```python
from build123d import *

# Parameters (mm, degrees)
SKETCH1_R             = 2
BOSS_EXTRUDE1_DEPTH   = 8
BOSS_EXTRUDE1_2_DEPTH = 8
BOSS_EXTRUDE2_DEPTH   = 20
BOSS_EXTRUDE3_DEPTH   = 20
BOSS_EXTRUDE4_START   = -8
SKETCH4_R             = 2
BOSS_EXTRUDE4_DEPTH   = 8
CUT_EXTRUDE1_DEPTH    = 133.91350571
SKETCH7_W             = 3
SKETCH7_H             = 9
BOSS_EXTRUDE5_DEPTH   = 20
BOSS_EXTRUDE6_DEPTH   = 3
CUT_EXTRUDE2_DEPTH    = 132.780119897
MIRROR2_COPY_1_DEPTH  = 3
MIRROR2_COPY_2_DEPTH  = 132.780119897
MIRROR3_COPY_1_DEPTH  = 3
MIRROR3_COPY_2_DEPTH  = 132.780119897
MIRROR3_COPY_3_DEPTH  = 3
MIRROR3_COPY_4_DEPTH  = 132.780119897
MIRROR3_COPY_5_DEPTH  = 3
MIRROR3_COPY_6_DEPTH  = 132.780119897


with BuildPart() as part:
    # Sketch1 → Boss-Extrude1 (new body)
    with BuildSketch(Plane.XY):
        with BuildLine():
            Line((-10, -15), (10, -15))
            ThreePointArc((10, -15), (0, -25), (-10, -15))
        make_face()
        with Locations((0, -19)):
            Circle(SKETCH1_R, mode=Mode.SUBTRACT)
    extrude(amount=-BOSS_EXTRUDE1_DEPTH)



with BuildPart() as body_2:
    # Sketch1 → Boss-Extrude1 2 (new body)
    with BuildSketch(Plane.XY):
        with BuildLine():
            Line((10, 0), (-10, 0))
            ThreePointArc((-10, 0), (0, 10), (10, 0))
        make_face()
        with Locations((0, 4)):
            Circle(SKETCH1_R, mode=Mode.SUBTRACT)
    extrude(amount=-BOSS_EXTRUDE1_2_DEPTH)


with BuildPart() as part_1:
    add(part.part)

    add(body_2.part)  # Boss-Extrude2 merges body 2
    # Sketch2 → Boss-Extrude2 (add)
    with BuildSketch(Plane.ZY.offset(10)):
        Polygon((0, -15), (67, -15), (67, -7.5), (54, -7.5), (54, 0), (0, 0), (-8, 0), (-8, -15), align=None)
    extrude(amount=-BOSS_EXTRUDE2_DEPTH)

    # Sketch3 → Boss-Extrude3 (add)
    with BuildSketch(Plane.ZY.offset(10)):
        Polygon((54, 0), (54, -7.5), (67, -7.5), (67, -15), (121, -15), (129, -15), (129, 0), (121, 0), align=None)
    extrude(amount=-BOSS_EXTRUDE3_DEPTH)

    # Sketch4 → Boss-Extrude4 (add)
    # profile 1 of 2: a face of its own
    with BuildSketch(Plane(origin=(0, 0, 121), x_dir=(-1, 0, 0), z_dir=(0, 0, -1)).offset(BOSS_EXTRUDE4_START)):
        with BuildLine():
            Line((-10, 0), (10, 0))
            ThreePointArc((10, 0), (0, 10), (-10, 0))
        make_face()
        with Locations(Location((0, 4, 0), (0, 0, 180))):
            Circle(SKETCH4_R, mode=Mode.SUBTRACT)
    # profile 2 of 2: a face of its own
    with BuildSketch(Plane(origin=(0, 0, 121), x_dir=(-1, 0, 0), z_dir=(0, 0, -1)).offset(BOSS_EXTRUDE4_START)):
        with BuildLine():
            Line((10, -15), (-10, -15))
            ThreePointArc((-10, -15), (0, -25), (10, -15))
        make_face()
        with Locations(Location((0, -19, 0), (0, 0, 180))):
            Circle(SKETCH4_R, mode=Mode.SUBTRACT)
    extrude(amount=BOSS_EXTRUDE4_DEPTH)

    # Sketch6 → Cut-Extrude1 (cut, through all)
    with BuildSketch(Plane(origin=(10, 0, 0), x_dir=(0, 0, -1), z_dir=(1, 0, 0))):
        Polygon((0, -3), (-121, -3), (-126, -3), (-126, -12), (-121, -12), (0, -12), (5, -12), (5, -3), align=None)
    extrude(amount=-CUT_EXTRUDE1_DEPTH, mode=Mode.SUBTRACT)

    # Sketch7 → Boss-Extrude5 (add)
    with BuildSketch(Plane(origin=(10, 0, 0), x_dir=(0, 0, -1), z_dir=(1, 0, 0))):
        Polygon((5, -12), (-8.403331864, -3), (-8.403331864, -4.806786238), (2.309227161, -12), align=None)
        Polygon((-5.712559024, -3), (-8.403331864, -3), (5, -12), (5, -10.193213762), align=None)
        Polygon((-11.403331864, -3), (-11.403331864, -12), (-8.403331864, -12), (-8.403331864, -4.806786238), (-8.403331864, -3), align=None)
        Polygon((-30.703894148, -3), (-37.802498898, -3), (-18.501936613, -12), (-11.403331864, -12), align=None)
        with Locations((-39.302498898, -7.5)):
            Rectangle(SKETCH7_W, SKETCH7_H)
        Polygon((-60.103061182, -3), (-67.201665932, -3), (-47.901103647, -12), (-40.802498898, -12), align=None)
        with Locations((-68.701665932, -7.5)):
            Rectangle(SKETCH7_W, SKETCH7_H)
        Polygon((-89.502228216, -3), (-96.600832966, -3), (-77.300270681, -12), (-70.201665932, -12), align=None)
        with Locations((-98.100832966, -7.5)):
            Rectangle(SKETCH7_W, SKETCH7_H)
        Polygon((-118.901395251, -3), (-126, -3), (-106.699437715, -12), (-99.600832966, -12), align=None)
    extrude(amount=-BOSS_EXTRUDE5_DEPTH)

    # Sketch9 → Boss-Extrude6 (add)
    with BuildSketch(Plane(origin=(5, 0, 0), x_dir=(0, 0, -1), z_dir=(1, 0, 0))):
        Polygon((0, -15), (0, -23.702060424), (-15, -15), align=None)
    boss_extrude6 = extrude(amount=BOSS_EXTRUDE6_DEPTH)

    # Sketch10 → Cut-Extrude2 (cut, through all)
    with BuildSketch(Plane(origin=(0, 0, 0), x_dir=(-1, 0, 0), z_dir=(0, 0, -1))):
        with BuildLine():
            Line((-8, -21), (-8, -23.702060424))
            Line((-8, -23.702060424), (-5, -23.702060424))
            Line((-5, -23.702060424), (-5, -23.660254038))
            ThreePointArc((-5, -23.660254038), (-6.634699532, -22.482029278), (-8, -21))
        make_face()
    cut_extrude2 = extrude(amount=-CUT_EXTRUDE2_DEPTH, mode=Mode.SUBTRACT)

    # Mirror1: Boss-Extrude6, Cut-Extrude2 across plane
    add(boss_extrude6.mirror(Plane(origin=(0, 0, 0), x_dir=(0, 0, 1), z_dir=(1, 0, 0))))
    add(cut_extrude2.mirror(Plane(origin=(0, 0, 0), x_dir=(0, 0, 1), z_dir=(1, 0, 0))), mode=Mode.SUBTRACT)

    # Mirror2: Boss-Extrude6, Cut-Extrude2 across plane
    add(boss_extrude6.mirror(Plane(origin=(0, 0, 60.5), x_dir=(1, 0, 0), z_dir=(0, 0, -1))))
    add(cut_extrude2.mirror(Plane(origin=(0, 0, 60.5), x_dir=(1, 0, 0), z_dir=(0, 0, -1))), mode=Mode.SUBTRACT)

    # Mirror2 copy 1 sketch → Mirror2 copy 1 (add)
    with BuildSketch(Plane(origin=(-5, 0, 121), x_dir=(0, 0, 1), z_dir=(-1, 0, 0))):
        Polygon((0, -15), (0, -23.702060424), (-15, -15), align=None)
    extrude(amount=MIRROR2_COPY_1_DEPTH)

    # Mirror2 copy 2 sketch → Mirror2 copy 2 (cut, through all)
    with BuildSketch(Plane.XY.offset(121)):
        with BuildLine():
            Line((-8, -21), (-8, -23.702060424))
            Line((-8, -23.702060424), (-5, -23.702060424))
            Line((-5, -23.702060424), (-5, -23.660254038))
            ThreePointArc((-5, -23.660254038), (-6.634699532, -22.482029278), (-8, -21))
        make_face()
    extrude(amount=-MIRROR2_COPY_2_DEPTH, mode=Mode.SUBTRACT)

    # Mirror3: Boss-Extrude6, Cut-Extrude2 across plane
    add(boss_extrude6.mirror(Plane.ZX.offset(-7.5)))
    add(cut_extrude2.mirror(Plane.ZX.offset(-7.5)), mode=Mode.SUBTRACT)

    # Mirror3 copy 1 sketch → Mirror3 copy 1 (add)
    with BuildSketch(Plane(origin=(-5, -15, 0), x_dir=(0, 0, -1), z_dir=(-1, 0, 0))):
        Polygon((0, -15), (0, -23.702060424), (-15, -15), align=None)
    extrude(amount=MIRROR3_COPY_1_DEPTH)

    # Mirror3 copy 2 sketch → Mirror3 copy 2 (cut, through all)
    with BuildSketch(Plane(origin=(0, -15, 0), x_dir=(1, 0, 0), z_dir=(0, 0, -1))):
        with BuildLine():
            Line((-8, -21), (-8, -23.702060424))
            Line((-8, -23.702060424), (-5, -23.702060424))
            Line((-5, -23.702060424), (-5, -23.660254038))
            ThreePointArc((-5, -23.660254038), (-6.634699532, -22.482029278), (-8, -21))
        make_face()
    extrude(amount=-MIRROR3_COPY_2_DEPTH, mode=Mode.SUBTRACT)

    # Mirror3 copy 3 sketch → Mirror3 copy 3 (add)
    with BuildSketch(Plane(origin=(5, -15, 121), x_dir=(0, 0, 1), z_dir=(1, 0, 0))):
        Polygon((0, -15), (0, -23.702060424), (-15, -15), align=None)
    extrude(amount=MIRROR3_COPY_3_DEPTH)

    # Mirror3 copy 4 sketch → Mirror3 copy 4 (cut, through all)
    with BuildSketch(Plane(origin=(0, -15, 121), x_dir=(-1, 0, 0), z_dir=(0, 0, 1))):
        with BuildLine():
            Line((-8, -21), (-8, -23.702060424))
            Line((-8, -23.702060424), (-5, -23.702060424))
            Line((-5, -23.702060424), (-5, -23.660254038))
            ThreePointArc((-5, -23.660254038), (-6.634699532, -22.482029278), (-8, -21))
        make_face()
    extrude(amount=-MIRROR3_COPY_4_DEPTH, mode=Mode.SUBTRACT)

    # Mirror3 copy 5 sketch → Mirror3 copy 5 (add)
    with BuildSketch(Plane(origin=(-5, -15, 121), x_dir=(0, 0, 1), z_dir=(-1, 0, 0))):
        Polygon((0, 15), (0, 23.702060424), (-15, 15), align=None)
    extrude(amount=MIRROR3_COPY_5_DEPTH)

    # Mirror3 copy 6 sketch → Mirror3 copy 6 (cut, through all)
    with BuildSketch(Plane(origin=(0, -15, 121), x_dir=(1, 0, 0), z_dir=(0, 0, 1))):
        with BuildLine():
            Line((-8, 21), (-8, 23.702060424))
            Line((-8, 23.702060424), (-5, 23.702060424))
            Line((-5, 23.702060424), (-5, 23.660254038))
            ThreePointArc((-5, 23.660254038), (-6.634699532, 22.482029278), (-8, 21))
        make_face()
    extrude(amount=-MIRROR3_COPY_6_DEPTH, mode=Mode.SUBTRACT)


solid = part_1.part
```
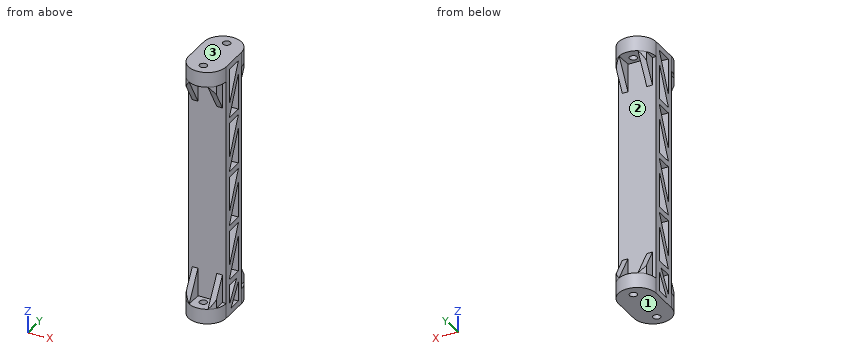
Read the model definition and answer for the solid it produces. Units are mm, in the model's axes. Face numbers are marked on the shaded views. Give positions to 0.01 mm unless a question says otherwise; leave off trailing zeros. Write each loop counter-clockwise with the first axis right and the second up, starting at its lowest first coordinate (ties: lowest second). Pieces come first, ordered by that corner, then holes. Notation, with made-up numbers: M 49.5,81.5 L 53.5,81.5 A21 cw 53.5,112.5 Z; hole C -19.5,-39.75 d4. An arc over 180 degrees is marked long. Put each result on its own line as item: value. Start each with the question number.
1. The part is cut by section C-C, the plane z = 79. Give the vertices of the cut face in (x, y).
2. Consider line 1 along Y through (x, z) = (0, 125); line 2 along Y through (x, z) = (0, 123.75); line 3 along Y through (x, z) = (-7.5, 115.5). Determine where each line is inside the solid, lowest interval first.
3. The part is cut by section A-A, the plane z = 62.5. Give the vertices of the cut face in (x, y), and give its area (3 significant figures).
4. The part is cut by section B-B, the plane y = 4. Give the number of separate pieces and of enclosed holes in the cut face, and give its area (3 significant figures).
5. The part is cut by section D-D, the plane z = 94.5. Give the vertices of the cut face in (x, y).
6. For a pull along Z with two mould halves and no side action, classify the marked faces 1, 2 and 3 as released by +Z, released by -Z, zero draft, split by the parting line, or undercut.
7. Each of these flat-tipped pins is pushed along its axis until it touches: pin 1 Ø3 at (y, z) = (2.5, 5) entering from +X; pin 2 Ø5 at (x, z) = (6.5, 28.5) entering from +Y. Where does it stop, or does it pass through?
Final values:
1. outline: M -10,-15 L 10,-15 L 10,-12 L -10,-12 Z; M -10,-11.21 L 10,-11.21 L 10,-7.9 L -10,-7.9 Z; M -10,-3 L 10,-3 L 10,0 L -10,0 Z
2. line 1: y = -25 to -21, -17 to -12, -3.47 to 2, 6 to 10
2. line 2: y = -25 to -21, -17 to -12, -4.05 to 2, 6 to 10
2. line 3: y = -20.51 to -12, -7.9 to -4.59, -3 to 5.51
3. outline: M -10,-15 L 10,-15 L 10,-12 L -10,-12 Z; M -10,-5.19 L 10,-5.19 L 10,0 L -10,0 Z
3. area: 164 mm²
4. separate pieces: 4
4. enclosed holes: 0
4. area: 327 mm²
5. outline: M -10,-15 L 10,-15 L 10,-12 L -10,-12 Z; M -10,-3.98 L 10,-3.98 L 10,0 L -10,0 Z
6. face 1: released by -Z
6. face 2: undercut
6. face 3: released by +Z
7. pin 1: stops at x = 8
7. pin 2: stops at y = 0
